Geometry check sheet. Reference: the model listing, model coordinates, mm. Face numbers are marked on the shaded views. A direction names the side the tool comes from. Coordinates: 2 decimals unless noted, no trailing zeros. Write each loop counter-clockwise with the first axis right and the second up, starting at its lowest first coordinate (ties: lowest second). Pieces come first, ordered by that corner, then holes. Notation, with made-up numbers: (57, -20.75) -> (68, -20.75) arc R21 cw to (68, -8.75) -> close; hole circle Ø3 at (-37, 77.5). An arc over 180 degrees is marked (long way). One line per question, with ' | ' between items.
from build123d import *

# Parameters (mm, degrees)
F1_DEPTH  = 76.2
F3_DEPTH  = 12.7
F2_W      = 38.1
F2_H      = 50.8
F4_DEPTH  = 25.4
F5_DEPTH  = 25.4
F6_R      = 12.7
F7_R      = 38.1
F8_DEPTH  = 25.4
F9_DEPTH  = 25.401
F10_DEPTH = 12.7


# Not quite as in the source:
# - a pattern or mirror of a feature is missing from the dataset's text; its kind, count and spacing are read off the source's solid
# - a feature names something its author has since deleted; it is built from what else it names


with BuildPart() as f1:
    # F0 (on Front) → F1 (new body, symmetric)
    with BuildSketch(Plane.XZ):
        Polygon((25.4, 203.2), (0, 203.2), (0, 0), (254, 0), (254, 12.7), (254, 25.4), (63.5, 25.4), (25.4, 25.4), (25.4, 76.2), align=None)
    extrude(amount=F1_DEPTH, both=True)

    # F2 (on face) → F3 (cut)
    with BuildSketch(Plane.XY.offset(25.4)):
        with BuildLine():
            Line((215.9, -12.7), (254, -12.7))
            Line((254, -12.7), (254, 12.7))
            Line((254, 12.7), (215.9, 12.7))
            ThreePointArc((215.9, 12.7), (203.2, 0), (215.9, -12.7))
        make_face()
    extrude(amount=-F3_DEPTH, mode=Mode.SUBTRACT)

    # F2 (on face) → F4 (join)
    with BuildSketch(Plane.XY.offset(25.4)):
        with BuildLine():
            Line((25.4, -76.2), (215.9, -76.2))
            Line((215.9, -76.2), (215.9, -25.4))
            Line((215.9, -25.4), (254, -25.4))
            Line((254, -25.4), (254, -12.7))
            Line((254, -12.7), (215.9, -12.7))
            ThreePointArc((215.9, -12.7), (203.2, 0), (215.9, 12.7))
            Line((215.9, 12.7), (254, 12.7))
            Line((254, 12.7), (254, 25.4))
            Line((254, 25.4), (215.9, 25.4))
            Line((215.9, 25.4), (215.9, 76.2))
            Line((215.9, 76.2), (25.4, 76.2))
            Line((25.4, 76.2), (25.4, -76.2))
        make_face()
        with BuildLine():
            ThreePointArc((177.8, -25.4), (190.5, -38.1), (177.8, -50.8))
            Line((177.8, -50.8), (101.6, -50.8))
            ThreePointArc((101.6, -50.8), (88.9, -38.1), (101.6, -25.4))
            Line((101.6, -25.4), (177.8, -25.4))
        make_face(mode=Mode.SUBTRACT)
        with Locations((234.95, -50.8)):
            Rectangle(F2_W, F2_H)
        with BuildLine():
            Line((101.6, -50.8), (177.8, -50.8))
            ThreePointArc((177.8, -50.8), (190.5, -38.1), (177.8, -25.4))
            Line((177.8, -25.4), (101.6, -25.4))
            ThreePointArc((101.6, -25.4), (88.9, -38.1), (101.6, -50.8))
        make_face()
    extrude(amount=-F4_DEPTH)

    # F2 (on face) → F5 (cut)
    with BuildSketch(Plane.XY.offset(25.4)):
        with Locations((234.95, -50.8)):
            Rectangle(F2_W, F2_H)
        with Locations((234.95, 50.8)):
            Rectangle(F2_W, F2_H)
    extrude(amount=-F5_DEPTH, mode=Mode.SUBTRACT)

    # F6
    f6_edges = [f1.edges().sort_by_distance(p)[0] for p in [
        (215.9, -25.4, 12.7),
        (215.9, -76.2, 12.7),
        (215.9, 25.4, 12.7),
        (215.9, 76.2, 12.7),
    ]]
    fillet(f6_edges, radius=F6_R)

    # F7 (on face) → F8 (cut)
    with BuildSketch(Plane(origin=(0, 0, 0), x_dir=(0, -1, 0), z_dir=(-1, 0, 0))):
        with BuildLine():
            ThreePointArc((3.576e-07, 203.2), (53.8815368528, 180.8815366), (76.2, 127))
            Line((76.2, 127), (76.2, 203.2))
            Line((76.2, 203.2), (3.576e-07, 203.2))
        make_face()
        with Locations((0, 127)):
            Circle(F7_R)
        with BuildLine():
            ThreePointArc((-76.2, 127), (-53.8815366, 180.8815368528), (3.576e-07, 203.2))
            Line((3.576e-07, 203.2), (-76.2, 203.2))
            Line((-76.2, 203.2), (-76.2, 127))
        make_face()
    extrude(amount=-F8_DEPTH, mode=Mode.SUBTRACT)

    # F2 (on face) → F9 (cut, through all)
    with BuildSketch(Plane.XY.offset(25.4)):
        with BuildLine():
            Line((101.6, -50.8), (177.8, -50.8))
            ThreePointArc((177.8, -50.8), (190.5, -38.1), (177.8, -25.4))
            Line((177.8, -25.4), (101.6, -25.4))
            ThreePointArc((101.6, -25.4), (88.9, -38.1), (101.6, -50.8))
        make_face()
    f9 = extrude(amount=-F9_DEPTH, mode=Mode.SUBTRACT)

    # F9_copies: F9 across plane
    add(f9.mirror(Plane.ZX), mode=Mode.SUBTRACT)

    # F0 (on Front) → F10 (join, symmetric)
    with BuildSketch(Plane.XZ):
        Polygon((63.5, 25.4), (25.4, 76.2), (25.4, 25.4), align=None)
    extrude(amount=F10_DEPTH, both=True)


solid = f1.part
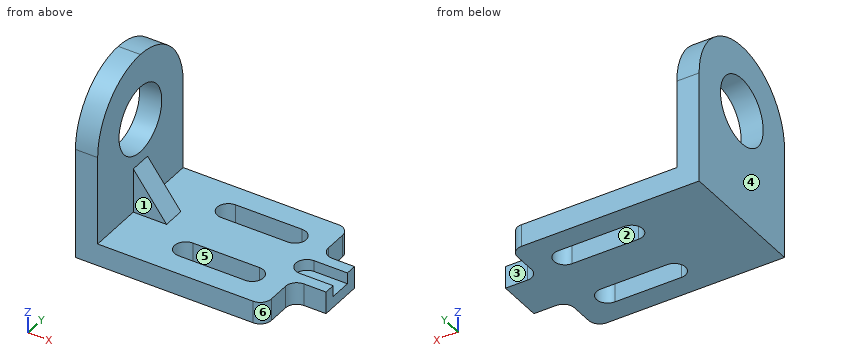
1. Cross-section at B-B on y = 4. Record the boundary of the cut face in (x, z).
Worked answers:
outline: (0, 0) -> (254, 0) -> (254, 12.7) -> (203.85, 12.7) -> (203.85, 25.4) -> (63.5, 25.4) -> (25.4, 76.2) -> (25.4, 89.11) -> (0, 89.11) -> close; (0, 164.89) -> (25.4, 164.89) -> (25.4, 203.09) -> (0, 203.09) -> close
2. Go/stop test with flat-tipped pins: P1, Ø10, axis at x = 226, y = -8, coming from the +Z side; P2, Ø6.5, axis at x = 233, z = 16.5, coming from the +Y side; P3, Ø7.5, axis at x = 244.5, z = 19, coming from the -Y side. Record where each tip stops, or that it passes through.
Worked answers:
P1: z = 25.4 | P2: y = 25.4 | P3: y = -25.4
3. Material ranges on line 1 (Z direction, x = 12, y = 0); line 2 (X direction, y = -61, z = 15); line 3 (X direction, y = 14.5, z = 68), recorded low to high. Write a range as from..to.
Worked answers:
line 1: 0..88.9, 165.1..203.2 | line 2: 0..215.9 | line 3: 0..25.4
4. Tool access check on the marked faces 1, 2 and 3. Record the directions out of +Z, -Z, +X, -X, +Y, -Y that give a thin tool (end or side, any length) a straight path to the whole face; none if there is none.
Worked answers:
face 1: +Z, +X, -Y | face 2: +Z, -Z | face 3: +Z, -Z, +X, +Y
5. Mould release check, pull along Y, two halves, no side actions. Record for the marked faces 4, 5 and 6: released by +Y, released by -Y, zero draft, split by the parting line, or undercut.
Worked answers:
face 4: zero draft | face 5: undercut | face 6: released by -Y
6. Cross-section at C-C on x = 60.5. Record the boundary of the cut face in (y, z), and give its area (3 significant figures).
Worked answers:
outline: (-76.2, 0) -> (76.2, 0) -> (76.2, 25.4) -> (12.7, 25.4) -> (12.7, 29.4) -> (-12.7, 29.4) -> (-12.7, 25.4) -> (-76.2, 25.4) -> close | area: 3,970 mm²
7. Cross-section at A-A on z = 20.5. Record the boundary of the cut face in (x, y).
Worked answers:
outline: (0, -76.2) -> (203.2, -76.2) arc R12.7 ccw to (215.9, -63.5) -> (215.9, -38.1) arc R12.7 cw to (228.6, -25.4) -> (254, -25.4) -> (254, -12.7) -> (215.9, -12.7) arc R12.7 cw to (215.9, 12.7) -> (254, 12.7) -> (254, 25.4) -> (228.6, 25.4) arc R12.7 cw to (215.9, 38.1) -> (215.9, 63.5) arc R12.7 ccw to (203.2, 76.2) -> (0, 76.2) -> close; hole (101.6, -50.8) -> (177.8, -50.8) arc R12.7 ccw to (177.8, -25.4) -> (101.6, -25.4) arc R12.7 ccw to start; hole (101.6, 25.4) -> (177.8, 25.4) arc R12.7 ccw to (177.8, 50.8) -> (101.6, 50.8) arc R12.7 ccw to start
8. Cross-section at D-D on y = 28.5. Record the boundary of the cut face in (x, z), and give its area (3 significant figures).
Worked answers:
outline: (0, 0) -> (93.29, 0) -> (93.29, 25.4) -> (25.4, 25.4) -> (25.4, 101.71) -> (0, 101.71) -> close; (0, 152.29) -> (25.4, 152.29) -> (25.4, 197.67) -> (0, 197.67) -> close; (186.11, 0) -> (220.29, 0) -> (220.29, 25.4) -> (186.11, 25.4) -> close | area: 6,330 mm²
